Work out the finished part from the listing and answer in its coordinate system (mm). Face numbers are marked on the shaded views. A direction names the side the tool comes from. Coordinates: 2 decimals unless noted, no trailing zeros. Order: outer loops, then holes, each group sorted by start corner. A loop starts at its lowest first (then second) coordinate and runs counter-clockwise, first axis right, second up.
1. The part is cut by section A-A, the plane x = 36. Give the vertices of the cut face in (y, z).
2. Determine the mould class of the marked faces 3, 4 and 5 for opening direction Y: +Y half, -Y half, draft (parallel to the pull), parting line (faces both ways), or undercut.
3. The part is cut by section D-D, the plane y = 34.5. Give the vertices of the cut face in (x, z), then the cut area to 3 significant figures.
4. Flat-ended cylindrical pins translate along their axes: pin 1 Ø1.2 at (x, y) = (43.75, -14.21) entering from +Z; pin 2 Ø6 at (x, z) = (15, 10.5) entering from -Y; pin 3 Ø2 at (x, z) = (30, 14.5) entering from -Y. Find the tip coordinate at first contact, or state that the pin passes through.
5. Find the intervals of material crossed by probe 1 along Y at (x, z) = (27, 15.5); probe 2 along Y at (x, z) = (-0.5, 6.5); probe 3 along Z at (x, y) = (37, 22), in increasing order.
6. The part is cut by section C-C, the plane y = -29.5. Give the vertices of the cut face in (x, z).
7. The part is cut by section B-B, the plane z = 15. Give the vertices of the cut face in (x, y), then the cut area to 3 significant figures.
8. A tool of negligible diameter and unlimited length cuts with its end or side. For the marked faces 1 and 2, from which of +Z, -Z, +X, -X, +Y, -Y can it reach the whole face along a straight path? Write none if from no direction.
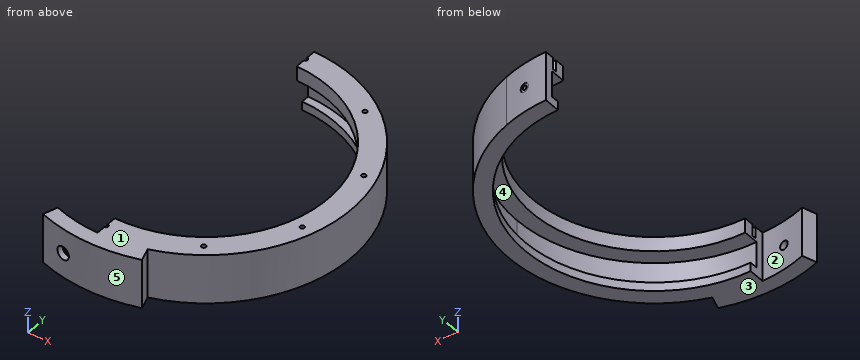
```python
from build123d import *

# Parameters (mm, degrees)
SKETCH_1_R               = 49.25
SKETCH_1_R_2             = 44.5
EXTRUDE_1_DEPTH          = 17
CUT_EXTRUDE_START        = 17
SKETCH_1_5_R             = 47.25
CUT_EXTRUDE_2_DEPTH      = 14
EXTRUDE_START            = 12
SKETCH_1_6_R             = 49.25
SKETCH_1_6_R_2           = 42
EXTRUDE_2_DEPTH          = 5
SKETCH_2_R               = 50
SKETCH_2_R_2             = 49.25
EXTRUDE_3_DEPTH          = 17
SKETCH_2_4_R             = 0.75
CUT_EXTRUDE_3_DEPTH      = 4
PATTERN_CIRCULAR_1_COUNT = 10
EXTRUDE_START_2          = 8.5
EXTRUDE_4_DEPTH          = 17
PATTERN_CIRCULAR_2_COUNT = 2
CUT_EXTRUDE_START_2      = -8.5
CUT_EXTRUDE_5_DEPTH      = 17


# Read off the part's stored shape, not the designer's step: 切除-拉伸5
with BuildPart() as part:
    # 草图1 → 凸台-拉伸1 (new body)
    with BuildSketch(Plane.XY):
        Circle(SKETCH_1_R)
        Circle(SKETCH_1_R_2, mode=Mode.SUBTRACT)
    extrude(amount=EXTRUDE_1_DEPTH)

    # 草图1<5> → 切除-拉伸2 (cut)
    with BuildSketch(Plane.XY.offset(CUT_EXTRUDE_START)):
        Circle(SKETCH_1_5_R)
    extrude(amount=-CUT_EXTRUDE_2_DEPTH, mode=Mode.SUBTRACT)

    # 草图1<6> → 凸台-拉伸2 (add)
    with BuildSketch(Plane.XY.offset(EXTRUDE_START)):
        Circle(SKETCH_1_6_R)
        Circle(SKETCH_1_6_R_2, mode=Mode.SUBTRACT)
    extrude(amount=EXTRUDE_2_DEPTH)

    # 草图2 → 凸台-拉伸3 (add, through all)
    with BuildSketch(Plane.XY.offset(17)):
        Circle(SKETCH_2_R)
        Circle(SKETCH_2_R_2, mode=Mode.SUBTRACT)
    extrude(amount=-EXTRUDE_3_DEPTH)

    # 草图2<4> → 切除-拉伸3 (cut)
    with BuildSketch(Plane.XY.offset(17)):
        with Locations((0, 46)):
            Circle(SKETCH_2_4_R)
    cut_extrude_3 = extrude(amount=-CUT_EXTRUDE_3_DEPTH, mode=Mode.SUBTRACT)

    # 阵列(圆周)1: 切除-拉伸3 ×10 about axis
    pattern_circular_1_axis = Axis((0, 0, 0), (0, 0, 1))
    for i in range(1, PATTERN_CIRCULAR_1_COUNT):
        add(cut_extrude_3.rotate(pattern_circular_1_axis, i * 360 / PATTERN_CIRCULAR_1_COUNT), mode=Mode.SUBTRACT)

    # 草图3 → 凸台-拉伸4 (add)
    with BuildSketch(Plane.XY.offset(8.5).offset(EXTRUDE_START_2)):
        with BuildLine():
            Line((15.450849719, 47.552825815), (16.995934691, 52.308108396))
            ThreePointArc((16.995934691, 52.308108396), (0, 55), (-16.995934691, 52.308108396))
            Line((-16.995934691, 52.308108396), (-15.450849719, 47.552825815))
            ThreePointArc((-15.450849719, 47.552825815), (0, 50), (15.450849719, 47.552825815))
        make_face()
    extrude_4 = extrude(amount=-EXTRUDE_4_DEPTH)

    # 草图3<5> → 切除-旋转1 (revolve, cut)
    with BuildSketch(Plane.XY.offset(8.5)):
        Polygon((6.324547295, 49.520299893), (7.06531355, 49.402974044), (7.806079806, 49.285648196), (8.291026647, 52.347482052), (6.809494136, 52.582133749), align=None)
        Polygon((7.806079806, 49.285648196), (7.06531355, 49.402974044), (6.43957569, 45.452220682), (7.180341945, 45.334894833), align=None)
        Polygon((6.809494136, 52.582133749), (8.291026647, 52.347482052), (8.603895577, 54.322858733), (6.381596811, 54.674836279), (6.068727881, 52.699459598), align=None)
    cut_revolve_1 = revolve(axis=Axis((7.821723252, 49.38441703, 8.5), (-0.15643446504023117, -0.9876883405951378, 0)), mode=Mode.SUBTRACT)

    # 阵列(圆周)2: 凸台-拉伸4, 切除-旋转1 ×2 about axis
    pattern_circular_2_axis = Axis((0, 0, 0), (0, 0, 1))
    add([extrude_4.rotate(pattern_circular_2_axis, i * 360 / PATTERN_CIRCULAR_2_COUNT) for i in range(1, PATTERN_CIRCULAR_2_COUNT)])
    add([cut_revolve_1.rotate(pattern_circular_2_axis, i * 360 / PATTERN_CIRCULAR_2_COUNT) for i in range(1, PATTERN_CIRCULAR_2_COUNT)], mode=Mode.SUBTRACT)

    # 切除-拉伸5 outline → 切除-拉伸5 (cut)
    with BuildSketch(Plane.XY.offset(8.5).offset(CUT_EXTRUDE_START_2)):
        with BuildLine():
            ThreePointArc((0, 50), (7.821723252, 49.38441703), (15.450849719, 47.552825815))
            Line((15.450849719, 47.552825815), (16.995934691, 52.308108396))
            ThreePointArc((16.995934691, 52.308108396), (0, 55), (-16.995934691, 52.308108396))
            Line((-16.995934691, 52.308108396), (-15.450849719, 47.552825815))
            ThreePointArc((-15.450849719, 47.552825815), (-50, 0), (-15.450849719, -47.552825815))
            ThreePointArc((-15.450849719, -47.552825815), (-7.821723252, -49.38441703), (0, -50))
            Line((0, -50), (0, -42))
            ThreePointArc((0, -42), (-42, 0), (0, 42))
            Line((0, 42), (0, 50))
        make_face()
    extrude(amount=CUT_EXTRUDE_5_DEPTH, mode=Mode.SUBTRACT)


solid = part.part
```
Geometry says:
1. outline: (-34.7, 0) - (-26.16, 0) - (-26.16, 3) - (-30.6, 3) - (-30.6, 12) - (-21.63, 12) - (-21.63, 17) - (-34.7, 17) - close; (21.63, 12) - (30.6, 12) - (30.6, 3) - (26.16, 3) - (26.16, 0) - (34.7, 0) - (34.7, 17) - (21.63, 17) - close
2. face 3: draft
2. face 4: undercut
2. face 5: -Y half
3. outline: (23.95, 12) - (32.28, 12) - (32.28, 3) - (28.11, 3) - (28.11, 0) - (36.19, 0) - (36.19, 17) - (23.95, 17) - close
3. area: 121 mm2
4. pin 1: stops at z = 13
4. pin 2: stops at y = -53.67
4. pin 3: stops at y = -40.73
5. probe 1: y = -42.08 to -37.96, -36.47 to -32.17, 32.17 to 36.47, 37.96 to 42.08
5. probe 2: y = -55 to -50
5. probe 3: z = 12 to 17
6. outline: (29.9, 12) - (36.91, 12) - (36.91, 3) - (33.32, 3) - (33.32, 0) - (40.37, 0) - (40.37, 17) - (29.9, 17) - close
7. outline: (-17, -52.31) arc R55 ccw to (17, -52.31) - (15.45, -47.55) arc R50 ccw to (0, 50) - (0, 46.75) arc R0.75 cw to (0, 45.25) - (0, 42) arc R42 cw to (0, -42) - (0, -45.25) arc R0.75 cw to (0, -46.75) - (0, -50) arc R50 cw to (-15.45, -47.55) - close; hole circle Ø1.5 at (27.04, -37.21); hole circle Ø1.5 at (27.04, 37.21); hole circle Ø1.5 at (43.75, -14.21); hole circle Ø1.5 at (43.75, 14.21)
7. area: 1,310 mm2
8. face 1: +Z, +X, -X, +Y, -Y
8. face 2: +Z, -Z, +Y
